Read the model definition and answer for the solid it produces. Units are mm, in the model's axes. A direction names the side the tool comes from. Coordinates: 2 decimals unless noted, no trailing zeros. Loops run counter-clockwise (first coordinate to the right, second up) from the corner with the lowest first, then second, coordinate; pieces in that order, holes last.
from build123d import *

# Parameters (mm, degrees)
BOSS_EXTRUDE1_DEPTH = 1
BOSS_EXTRUDE2_START = 63.399999946
BOSS_EXTRUDE2_DEPTH = 63.399999946


with BuildPart() as part:
    # Sketch3 → Boss-Extrude1 (new body)
    with BuildSketch(Plane(origin=(0, 0, 0), x_dir=(1, 0, 0), z_dir=(0, 1, 0))):
        with BuildLine():
            Line((-117.504462868, 326.155640462), (-111.509184915, 332.971148344))
            ThreePointArc((-111.509184915, 332.971148344), (0, 384.155640476), (111.509184915, 332.971148344))
            Line((111.509184915, 332.971148344), (117.504462868, 326.155640462))
            Line((117.504462868, 326.155640462), (-117.504462868, 326.155640462))
        make_face()
    extrude(amount=BOSS_EXTRUDE1_DEPTH)

    # Sketch4 → Boss-Extrude2 (add)
    with BuildSketch(Plane.XZ.offset(BOSS_EXTRUDE2_START)):
        with BuildLine():
            Line((-117.504462868, -326.155640462), (-111.509184915, -332.971148344))
            ThreePointArc((-111.509184915, -332.971148344), (0, -384.155640476), (111.509184915, -332.971148344))
            Line((111.509184915, -332.971148344), (117.504462868, -326.155640462))
            Line((117.504462868, -326.155640462), (114.84078994, -326.155640462))
            Line((114.84078994, -326.155640462), (110, -331.658711753))
            ThreePointArc((110, -331.658711753), (0, -382.155640476), (-110, -331.658711753))
            Line((-110, -331.658711753), (-114.84078994, -326.155640462))
            Line((-114.84078994, -326.155640462), (-117.504462868, -326.155640462))
        make_face()
    extrude(amount=-BOSS_EXTRUDE2_DEPTH)


solid = part.part
Item 1: A cutting plane is placed at C-C on x = 14.5. Determine the outline of the cut face in (y, z), then the cut area to 3 significant figures.
Numbers:
outline: (-63.4, -383.44) - (1, -383.44) - (1, -326.16) - (0, -326.16) - (0, -381.43) - (-63.4, -381.43) - close
area: 185 mm2
Item 2: A cutting plane is placed at B-B on z = -373. Determine the outline of the cut face in (x, y).
Numbers:
outline: (-56.18, -63.4) - (-50.72, -63.4) - (-50.72, 0) - (50.72, 0) - (50.72, -63.4) - (56.18, -63.4) - (56.18, 1) - (-56.18, 1) - close
Item 3: A cutting plane is placed at D-D on x = 59.5. Determine the outline of the cut face in (y, z).
Numbers:
outline: (-63.4, -371.58) - (1, -371.58) - (1, -326.16) - (0, -326.16) - (0, -369.39) - (-63.4, -369.39) - close
Item 4: Find the intervals of material crossed by line 1 along Y through (x, z) = (-38, -352.5); line 2 along X through (y, z) = (-9.5, -339); line 3 along X through (y, z) = (-38.5, -356), in increasing order.
Numbers:
line 1: y = 0 to 1
line 2: x = -106.03 to -103.24, 103.24 to 106.03
line 3: x = -86.53 to -83.09, 83.09 to 86.53
Item 5: Determine the mould class of faces 1 (the face through (-114.549, -31.651, -329.516)), 2 (the face through (2, 1, -349)), 3 (the face through (1.748, -32.144, -382.145)), 4 (the face through (112.454, -32.144, -328.869)) for opening direction X: released by +X, released by -X, zero draft, split by the parting line, or undercut.
Numbers:
face 1: released by -X
face 2: zero draft
face 3: undercut
face 4: undercut
Item 6: Given pin 1 (4 mm diameter, centred on x = -55.5, z = -374, fed in from +Y); pin 2 (10 mm diameter, centred on y = -32, z = -350, fed in from +X); pin 3 (6 mm diameter, centred on y = -34, z = -376, fed in from +X); pin 4 (8 mm diameter, centred on x = -55.5, y = -10, fed in from +Z), each flat-ended and moving along its own axis, determine where each tip first touches the part or whether it passes through.
Numbers:
pin 1: stops at y = 1
pin 2: stops at x = 99.92
pin 3: stops at x = 56.18
pin 4: stops at z = -369.39
Item 7: A cutting plane is placed at A-A on y = -45. Determine the outline of the cut face in (x, z), then the cut area to 3 significant figures.
Numbers:
outline: (-117.5, -326.16) - (-111.51, -332.97) arc R147.06 ccw to (111.51, -332.97) - (117.5, -326.16) - (114.84, -326.16) - (110, -331.66) arc R145.06 cw to (-110, -331.66) - (-114.84, -326.16) - close
area: 536 mm2
Item 8: Which of the six approach directions +Z, -Z, +X, -X, +Y, -Y give full straight-line access (tool end or side, diameter ignored) to faces 5 (the face through (-1, -63.4, -383)), 6 (the face through (-112.387, -32.144, -328.946))?
Numbers:
face 5: +Z, -Z, +X, -X, -Y
face 6: +Z, -Y
